from build123d import *

# Parameters (mm, degrees)
SKETCH1_W           = 106
SKETCH1_H           = 60
BOSS_EXTRUDE1_DEPTH = 10
SKETCH2_W           = 10
SKETCH2_H           = 60
BOSS_EXTRUDE2_DEPTH = 55
SKETCH3_W           = 60
SKETCH3_H           = 15
BOSS_EXTRUDE3_DEPTH = 20
SKETCH4_W           = 60
SKETCH4_H           = 15
BOSS_EXTRUDE4_DEPTH = 20
SKETCH5_R           = 4.5
CUT_EXTRUDE1_DEPTH  = 66
SKETCH6_R           = 6.5
CUT_EXTRUDE2_DEPTH  = 6.6
SKETCH7_R           = 3.3
CUT_EXTRUDE3_DEPTH  = 9.4
FILLET1_R           = 1


with BuildPart() as part:
    # Sketch1 → Boss-Extrude1 (new body)
    with BuildSketch(Plane(origin=(0, 0, 0), x_dir=(1, 0, 0), z_dir=(0, 1, 0))):
        Rectangle(SKETCH1_W, SKETCH1_H)
    extrude(amount=BOSS_EXTRUDE1_DEPTH)

    # Sketch2 → Boss-Extrude2 (add)
    with BuildSketch(Plane.XZ):
        with Locations((-48, 0)):
            Rectangle(SKETCH2_W, SKETCH2_H)
        with Locations((48, 0)):
            Rectangle(SKETCH2_W, SKETCH2_H)
    extrude(amount=BOSS_EXTRUDE2_DEPTH)

    # Sketch3 → Boss-Extrude3 (add)
    with BuildSketch(Plane(origin=(53, 0, 0), x_dir=(0, 0, -1), z_dir=(1, 0, 0))):
        with Locations((0, -47.5)):
            Rectangle(SKETCH3_W, SKETCH3_H)
    extrude(amount=BOSS_EXTRUDE3_DEPTH)

    # Sketch4 → Boss-Extrude4 (add)
    with BuildSketch(Plane.ZY.offset(53)):
        with Locations((0, -47.5)):
            Rectangle(SKETCH4_W, SKETCH4_H)
    extrude(amount=BOSS_EXTRUDE4_DEPTH)

    # Sketch5 → Cut-Extrude1 (cut, through all)
    with BuildSketch(Plane(origin=(0, 10, 0), x_dir=(1, 0, 0), z_dir=(0, 1, 0))):
        with Locations((-32, 21)):
            Circle(SKETCH5_R)
        with Locations((32, 21)):
            Circle(SKETCH5_R)
        with Locations((32, -21)):
            Circle(SKETCH5_R)
        with Locations((-32, -21)):
            Circle(SKETCH5_R)
    extrude(amount=-CUT_EXTRUDE1_DEPTH, mode=Mode.SUBTRACT)

    # Sketch6 → Cut-Extrude2 (cut)
    with BuildSketch(Plane(origin=(0, -40, 0), x_dir=(1, 0, 0), z_dir=(0, 1, 0))):
        with Locations((63, 20)):
            Circle(SKETCH6_R)
        with Locations((63, -20)):
            Circle(SKETCH6_R)
        with Locations((-63, 20)):
            Circle(SKETCH6_R)
        with Locations((-63, -20)):
            Circle(SKETCH6_R)
    extrude(amount=-CUT_EXTRUDE2_DEPTH, mode=Mode.SUBTRACT)

    # Sketch7 → Cut-Extrude3 (cut, through all)
    with BuildSketch(Plane(origin=(0, -46.6, 0), x_dir=(1, 0, 0), z_dir=(0, 1, 0))):
        with Locations((-63, 20)):
            Circle(SKETCH7_R)
        with Locations((-63, -20)):
            Circle(SKETCH7_R)
        with Locations((63, -20)):
            Circle(SKETCH7_R)
        with Locations((63, 20)):
            Circle(SKETCH7_R)
    extrude(amount=-CUT_EXTRUDE3_DEPTH, mode=Mode.SUBTRACT)

    # Fillet1
    fillet1_edges = [part.edges().sort_by_distance(p)[0] for p in [
        (-43, -27.5, -30),
        (-43, -27.5, 30),
        (43, -27.5, 30),
        (43, -27.5, -30),
        (73, -47.5, 30),
        (73, -47.5, -30),
        (-73, -47.5, -30),
        (-73, -47.5, 30),
    ]]
    fillet(fillet1_edges, radius=FILLET1_R)


solid = part.part
Work out the finished part from the listing and answer in its coordinate system (mm). A direction names the side the tool comes from. Round coordinates to 2 decimals unless told otherwise and drop trailing zeros. Write each loop counter-clockwise with the first axis right and the second up, starting at its lowest first coordinate (ties: lowest second). Pieces come first, ordered by that corner, then holes.
1) The mould has two halves that part along Z. Classify faces 5 (the flat face through (-43, -27, 0)), 6 (the flat face through (-10, 1, -30)), 7 (the flat face through (-66, -46.6, 18)): pulls with the +Z half, pulls with the -Z half, needs draft (parallel to the pull), parting line crosses it, or undercut.
2) A cutting plane is placed at B-B (x = 32). Give the vertices of the cut face in (y, z).
3) Given pin 1 Ø2 at (y, z) = (-28.5, 9) entering from +X; pin 2 Ø10.5 at (x, z) = (63, 20) entering from +Y; pin 3 Ø10.5 at (x, z) = (-64.5, 23) entering from +Y, each flat-ended and moving along its own axis, determine where each tip first touches the part or whether it passes through.
4) A cutting plane is placed at D-D (y = -31). Give the vertices of the cut face in (x, z).
5) A cutting plane is placed at C-C (z = -4.5). Give the vertices of the cut face in (x, y), plus the area to 3 significant figures.
6) A cutting plane is placed at A-A (y = -51). Give the vertices of the cut face in (x, z), plus the area to 3 significant figures.
7) A tool of negligible diameter and unlimited length cuts with its end or side. For faces 1 (the flat face through (53, -15, 0)), 2 (the flat face through (-63, -40, 0)), 3 (the cylindrical face through (69.2, -43.25, 18.05)), 4 (the flat face through (43, -27, 0)), from which of +Z, -Z, +X, -X, +Y, -Y can it reach the whole face along a straight path? Write none if from no direction.
8) Straight lines are drawn through the part: line 1 (X direction, y = -49.5, z = -20); line 2 (Z direction, x = -63, y = -48.75); line 3 (X direction, y = 2, z = -21). For each, find the intervals that lie inside material, in ascending order.
Completed:
1. face 5: needs draft
1. face 6: pulls with the -Z half
1. face 7: undercut
2. outline: (0, -30) - (10, -30) - (10, -25.5) - (0, -25.5) - close; (0, -16.5) - (10, -16.5) - (10, 16.5) - (0, 16.5) - close; (0, 25.5) - (10, 25.5) - (10, 30) - (0, 30) - close
3. pin 1: stops at x = 53
3. pin 2: stops at y = -46.6
3. pin 3: stops at y = -40
4. outline: (-53, -30) - (-44, -30) arc R1 ccw to (-43, -29) - (-43, 29) arc R1 ccw to (-44, 30) - (-53, 30) - close; (43, -29) arc R1 ccw to (44, -30) - (53, -30) - (53, 30) - (44, 30) arc R1 ccw to (43, 29) - close
5. outline: (-73, -55) - (-43, -55) - (-43, 0) - (43, 0) - (43, -55) - (73, -55) - (73, -40) - (53, -40) - (53, 10) - (-53, 10) - (-53, -40) - (-73, -40) - close
5. area: 2,760 mm2
6. outline: (-73, -29) arc R1 ccw to (-72, -30) - (-44, -30) arc R1 ccw to (-43, -29) - (-43, 29) arc R1 ccw to (-44, 30) - (-72, 30) arc R1 ccw to (-73, 29) - close; (43, -29) arc R1 ccw to (44, -30) - (72, -30) arc R1 ccw to (73, -29) - (73, 29) arc R1 ccw to (72, 30) - (44, 30) arc R1 ccw to (43, 29) - close; hole circle Ø6.6 at (-63, -20); hole circle Ø6.6 at (-63, 20); hole circle Ø6.6 at (63, -20); hole circle Ø6.6 at (63, 20)
6. area: 3,460 mm2
7. face 1: +Z, -Z, +X, +Y
7. face 2: +Z, -Z, -X, +Y
7. face 3: +Y
7. face 4: +Z, -Z, -Y
8. line 1: x = -73 to -66.3, -59.7 to -43, 43 to 59.7, 66.3 to 73
8. line 2: z = -30 to -23.3, -16.7 to 16.7, 23.3 to 30
8. line 3: x = -53 to -36.5, -27.5 to 27.5, 36.5 to 53
